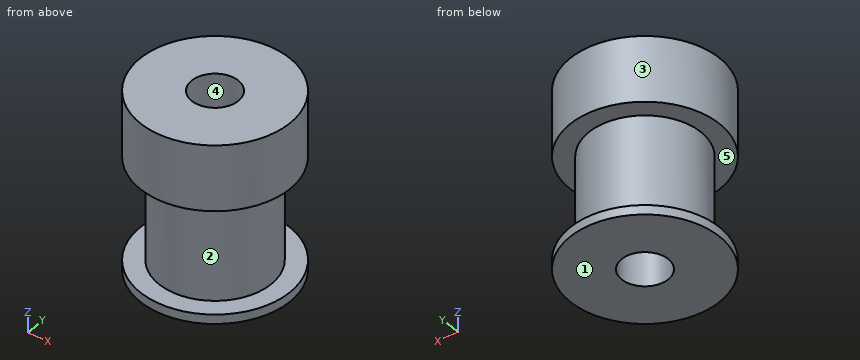
from build123d import *

# Parameters (mm, degrees)
SKETCH_1_R          = 8
EXTRUDE_1_DEPTH     = 19
CUT_EXTRUDE_START   = -18
SKETCH_2_R          = 8
SKETCH_2_R_2        = 6
CUT_EXTRUDE_3_DEPTH = 11
SKETCH_3_R          = 2.5
CUT_EXTRUDE_4_DEPTH = 23.113344387


with BuildPart() as part:
    # 草图1 → 凸台-拉伸1 (new body)
    with BuildSketch(Plane.XY):
        Circle(SKETCH_1_R)
    extrude(amount=EXTRUDE_1_DEPTH)

    # 草图2 → 切除-拉伸3 (cut)
    with BuildSketch(Plane.XY.offset(19).offset(CUT_EXTRUDE_START)):
        Circle(SKETCH_2_R)
        Circle(SKETCH_2_R_2, mode=Mode.SUBTRACT)
    extrude(amount=CUT_EXTRUDE_3_DEPTH, mode=Mode.SUBTRACT)

    # 草图3 → 切除-拉伸4 (cut, through all)
    with BuildSketch(Plane.XY.offset(19)):
        Circle(SKETCH_3_R)
    extrude(amount=-CUT_EXTRUDE_4_DEPTH, mode=Mode.SUBTRACT)


solid = part.part
Design review of the part built by this model. Coordinates are the model's own, in mm. Face numbers are marked on the shaded views. A direction names the side the tool comes from. Give positions to 0.01 mm unless a question says otherwise; leave off trailing zeros. Loops run counter-clockwise (first coordinate to the right, second up) from the corner with the lowest first, then second, coordinate; pieces in that order, holes last. Notation, with made-up numbers: M -20.75,85 L -13.75,85 A15 cw -13.75,108 Z; hole C 41.25,59 d4. An arc over 180 degrees is marked long. Answer as a JSON object with one key per item and string values.
Item 1: We need section D-D (y = -3.5). State the section outline as (x, z) points.
Output values:
{"outline": "M -7.19,0 L 7.19,0 L 7.19,1 L 4.87,1 L 4.87,12 L 7.19,12 L 7.19,19 L -7.19,19 L -7.19,12 L -4.87,12 L -4.87,1 L -7.19,1 Z"}
Item 2: For P1, Ø3, axis at x = 4, z = 6.5, coming from the +Y side; P2, Ø1, axis at x = 1, z = 2, coming from the -Y side; P3, Ø1, axis at x = -2, z = 6, coming from the -Y side, all flat-tipped, find the tip position at first contact; note any pin that passes through.
Output values:
{"P1": "stops at y = 5.45", "P2": "stops at y = -5.98", "P3": "stops at y = -5.81"}
Item 3: We need section A-A (y = 0). State the section outline as (x, z) points.
Output values:
{"outline": "M -8,0 L -2.5,0 L -2.5,19 L -8,19 L -8,12 L -6,12 L -6,1 L -8,1 Z; M 2.5,0 L 8,0 L 8,1 L 6,1 L 6,12 L 8,12 L 8,19 L 2.5,19 Z"}
Item 4: We need section C-C (z = 1.5). State the section outline as (x, y) points, and give its area (3 significant figures).
Output values:
{"outline": "C 0,0 d12; hole C 0,0 d5", "area": "93.5 mm2"}
Item 5: Machinability: for the marked faces 4 and 5, which of the approach directions +Z, -Z, +X, -X, +Y, -Y give a long, thin tool a straight path to every point of the face, cutting with its end or side? Answer none if there is none.
Output values:
{"face 4": "+Z, -Z", "face 5": "none"}
Item 6: Mouldability with a two-part tool opening along Z and no side actions: class the marked faces 1, 2 and 3 as pulls with the +Z half, pulls with the -Z half, needs draft (parallel to the pull), parting line crosses it, or undercut.
Output values:
{"face 1": "pulls with the -Z half", "face 2": "undercut", "face 3": "needs draft"}
Item 7: Wall thickness on line 1 along Z through (x, y) = (-1.75, -7); line 2 along Y through (x, z) = (0, 7.25); line 3 along X through (y, z) = (0.5, 16.5): over which ranges is each line inside the solid? List them lowest first.
Output values:
{"line 1": "z = 0 to 1, 12 to 19", "line 2": "y = -6 to -2.5, 2.5 to 6", "line 3": "x = -7.98 to -2.45, 2.45 to 7.98"}
